```python
from build123d import *

# Parameters (mm, degrees)
SKETCH1_R           = 7.3025
BOSS_EXTRUDE1_DEPTH = 165.1
SKETCH2_W           = 1.5875
SKETCH2_H           = 1.5875
SKETCH4_R           = 7.3025
SKETCH4_R_2         = 5.715
CUT_EXTRUDE1_DEPTH  = 1.6002
SKETCH5_OUTSIDE_W   = 49.882
SKETCH5_OUTSIDE_H   = 49.882
CUT_EXTRUDE2_DEPTH  = 12.7


with BuildPart() as part:
    # Sketch1 → Boss-Extrude1 (new body)
    with BuildSketch(Plane(origin=(0, 0, 0), x_dir=(0, 0, -1), z_dir=(1, 0, 0))):
        Circle(SKETCH1_R)
    extrude(amount=BOSS_EXTRUDE1_DEPTH)

    # Sketch2 → Groove (revolve, cut)
    with BuildSketch(Plane.XY, mode=Mode.PRIVATE) as groove_sk:
        with Locations((13.49375, 6.50875)):
            Rectangle(SKETCH2_W, SKETCH2_H)
    revolve(groove_sk.sketch.rotate(Axis((0, 0, 0), (1, 0, 0)), 90), axis=Axis((0, 0, 0), (1, 0, 0)), mode=Mode.SUBTRACT)

    # Sketch4 → Cut-Extrude1 (cut)
    with BuildSketch(Plane.ZY.offset(-141.2875)):
        Circle(SKETCH4_R)
        Circle(SKETCH4_R_2, mode=Mode.SUBTRACT)
    extrude(amount=-CUT_EXTRUDE1_DEPTH, mode=Mode.SUBTRACT)

    # Sketch5 outside → Cut-Extrude2 (cut)
    with BuildSketch(Plane(origin=(165.1, 0, 0), x_dir=(0, 0, -1), z_dir=(1, 0, 0))):
        Rectangle(SKETCH5_OUTSIDE_W, SKETCH5_OUTSIDE_H)
        Polygon((7.3025, 0), (3.65125, 6.324150511), (-3.65125, 6.324150511), (-7.3025, 0), (-3.65125, -6.324150511), (3.65125, -6.324150511), align=None, mode=Mode.SUBTRACT)
    extrude(amount=-CUT_EXTRUDE2_DEPTH, mode=Mode.SUBTRACT)


solid = part.part
```
Verification items for the finished model (mm, model axes). A direction names the side the tool comes from. Coordinates: 2 decimals unless noted, no trailing zeros. Loops run counter-clockwise (first coordinate to the right, second up) from the corner with the lowest first, then second, coordinate; pieces in that order, holes last. Notation, with made-up numbers: (-13, 53.5) -> (23, 53.5) arc R11 ccw to (23, 58.5) -> close; hole circle Ø5 at (49.5, -7). An arc over 180 degrees is marked (long way). Put each result on its own line as item: value.
1. Mould release check, pull along X, two halves, no side actions. Record for faces 1 (the face through (152.4, -3, 6)), 2 (the face through (142.888, -6, 0)), 3 (the face through (12.7, 6, 0)), 4 (the face through (6.26, 4.94, 5.38)): pulls with the +X half, pulls with the -X half, needs draft (parallel to the pull), parting line crosses it, or undercut.
Result set:
face 1: pulls with the +X half
face 2: undercut
face 3: undercut
face 4: needs draft
2. Section check B-B, the plane y = -3. Record the boundary of the cut face in (x, z).
Result set:
outline: (0, -6.66) -> (12.7, -6.66) -> (12.7, -4.86) -> (14.29, -4.86) -> (14.29, -6.66) -> (141.29, -6.66) -> (141.29, -4.86) -> (142.89, -4.86) -> (142.89, -6.66) -> (152.4, -6.66) -> (152.4, -5.57) -> (165.1, -5.57) -> (165.1, 5.57) -> (152.4, 5.57) -> (152.4, 6.66) -> (142.89, 6.66) -> (142.89, 4.86) -> (141.29, 4.86) -> (141.29, 6.66) -> (14.29, 6.66) -> (14.29, 4.86) -> (12.7, 4.86) -> (12.7, 6.66) -> (0, 6.66) -> close
3. Tool access check on faces 5 (the face through (159, -6.324, 0)), 6 (the face through (13.505, 3.477, -4.535)), 7 (the face through (152.4, 3, -6)), 8 (the face through (152.4, 3, 6)). Record the directions out of +Z, -Z, +X, -X, +Y, -Y that give a thin tool (end or side, any length) a straight path to the whole face; none if there is none.
Result set:
face 5: +Z, -Z, +X, -Y
face 6: none
face 7: -Z, +X, +Y
face 8: +Z, +X, +Y
4. Thickness scan on line 1 (X direction, y = 4, z = 4.75); line 2 (X direction, y = -6.5, z = -0.5); line 3 (Z direction, x = 55, y = -0.25). Record the ranges inside material, lowest first.
Result set:
line 1: x = 0 to 12.7, 14.29 to 141.29, 142.89 to 165.1
line 2: x = 0 to 12.7, 14.29 to 141.29, 142.89 to 152.4
line 3: z = -7.3 to 7.3
5. Section check A-A, the plane x = 154. Record the boundary of the cut face in (y, z), then the cut area to 3 significant figures.
Result set:
outline: (-6.32, -3.65) -> (0, -7.3) -> (6.32, -3.65) -> (6.32, 3.65) -> (0, 7.3) -> (-6.32, 3.65) -> close
area: 139 mm^2
6. Gauge pin test, flat ends, axial feed: P1, Ø8, axis at x = 159, z = 0, coming from the -Y side; P2, Ø1.1, axis at y = -7, z = 1, coming from the +X side; P3, Ø6, axis at x = 155.5, z = 0.5, coming from the +Y side. Record the tip position at first contact, or that the pin passes through.
Result set:
P1: stops at y = -6.32
P2: stops at x = 152.4
P3: stops at y = 6.32
7. Section check C-C, the plane x = 91. Record the boundary of the cut face in (y, z) (1 decimal), then the cut area to 3 significant figures.
Result set:
outline: circle Ø14.6 at (0, 0)
area: 168 mm^2
